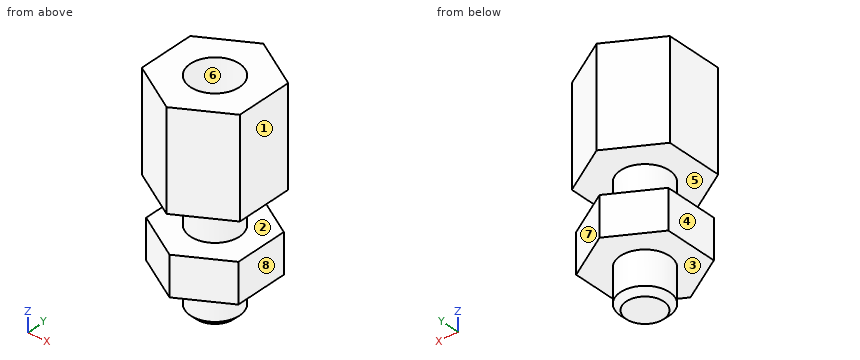
from build123d import *

# Parameters (mm, degrees)
F1_DEPTH = 5
F2_R     = 1.25
F3_DEPTH = 6
F4_R     = 1.25
F5_DEPTH = 2.5
F6_SIZE  = 0.3
F8_R     = 1.25
F9_DEPTH = 2


with BuildPart() as f1:
    # F0 (on Top) → F1 (new body)
    with BuildSketch(Plane.XY):
        Polygon((2.5, 1.443376), (0, 2.886751), (-2.5, 1.443376), (-2.5, -1.443376), (0, -2.886751), (2.5, -1.443376), align=None)
    extrude(amount=-F1_DEPTH)

    # F2 (on face) → F3 (join)
    with BuildSketch(Plane(origin=(0, 0, -5), x_dir=(1, 0, 0), z_dir=(0, 0, -1))):
        Circle(F2_R)
    extrude(amount=F3_DEPTH)

    # F4 (on face) → F5 (cut)
    with BuildSketch(Plane.XY):
        Circle(F4_R)
    extrude(amount=-F5_DEPTH, mode=Mode.SUBTRACT)

    # F6
    f6_edges = [f1.edges().sort_by_distance(p)[0] for p in [
        (-1.25, 0, -11),
    ]]
    chamfer(f6_edges, length=F6_SIZE)

    # F8 (on offset) → F9 (join)
    with BuildSketch(Plane(origin=(0, 0, -7), x_dir=(1, 0, 0), z_dir=(0, 0, -1))):
        Polygon((0, 2.713546), (-2.35, 1.356773), (-2.35, -1.356773), (0, -2.713546), (2.35, -1.356773), (2.35, 1.356773), align=None)
        Circle(F8_R, mode=Mode.SUBTRACT)
    extrude(amount=F9_DEPTH)


solid = f1.part
Could you check a few things on this model? Use its own coordinates, in mm. Face numbers are marked on the shaded views. A direction names the side the tool comes from. Coordinates: 2 decimals unless noted, no trailing zeros. Order: outer loops, then holes, each group sorted by start corner. A loop starts at its lowest first (then second) coordinate and runs counter-clockwise, first axis right, second up. Notation, with made-up numbers: (30.25, 12.25) -> (37.25, 12.25) arc R23 ccw to (37.25, 29.25) -> close; hole circle Ø3 at (88.5, -1). An arc over 180 degrees is marked (long way). One line per question, with ' | ' between items.
Q1. If I drill on L1, parallel to Z at x = 0.2, y = 1.3; L2, parallel to Y at x = 0.3, z = -4.5; L3, parallel to Z at x = -0.1, y = 0.05, over which ranges is the centre line in solid material (lowest first)?
Return value:
L1: -9 to -7, -5 to 0 | L2: -2.71 to 2.71 | L3: -11 to -2.5
Q2. Imagine slicing it at B-B on z = -7.5. Please give me the cut outline in (x, y), and give its area (3 significant figures).
Return value:
outline: (-2.35, -1.36) -> (0, -2.71) -> (2.35, -1.36) -> (2.35, 1.36) -> (0, 2.71) -> (-2.35, 1.36) -> close | area: 19.1 mm²
Q3. Imagine slicing it at C-C on y = 0. Please give me the cut outline in (x, z), and give its area (3 significant figures).
Return value:
outline: (-2.5, -5) -> (-1.25, -5) -> (-1.25, -7) -> (-2.35, -7) -> (-2.35, -9) -> (-1.25, -9) -> (-1.25, -10.7) -> (-0.95, -11) -> (0.95, -11) -> (1.25, -10.7) -> (1.25, -9) -> (2.35, -9) -> (2.35, -7) -> (1.25, -7) -> (1.25, -5) -> (2.5, -5) -> (2.5, 0) -> (1.25, 0) -> (1.25, -2.5) -> (-1.25, -2.5) -> (-1.25, 0) -> (-2.5, 0) -> close | area: 38.1 mm²
Q4. Imagine slicing it at A-A on y = -2.4. Please give me the cut outline in (x, z).
Return value:
outline: (-0.84, -5) -> (0.84, -5) -> (0.84, 0) -> (-0.84, 0) -> close; (-0.54, -9) -> (0.54, -9) -> (0.54, -7) -> (-0.54, -7) -> close
Q5. I'm going to push flat-ended pins straight in: P1, Ø1.6, axis at y = 0, z = -8.5, coming from the -X side; P2, Ø0.8, axis at x = -0.5, y = 0.5, coming from the +Z side; P3, Ø2, axis at y = 0, z = -9, coming from the +X side. Where does each tip first touch, or does it pass through?
Return value:
P1: x = -2.35 | P2: z = -2.5 | P3: x = 2.35
Q6. Thinking about a two-plate mould opening in Z: for the marked faces 1, 2 and 3, which applies, pulls with the +Z half, pulls with the -Z half, needs draft (parallel to the pull), parting line crosses it, or undercut?
Return value:
face 1: needs draft | face 2: undercut | face 3: pulls with the -Z half
Q7. On a 3-axis mill with a long thin cutter (end or side, diameter ignored), from which of +Z, -Z, +X, -X, +Y, -Y can I reach the whole of each face in a straight line? I mean the marked faces 4, 5, 6, 7 and 8. Say none if no direction works.
Return value:
face 4: -Z, -X, +Y, -Y | face 5: none | face 6: +Z | face 7: -Z, +X, +Y | face 8: -Z, +X, +Y, -Y
Q8. Imagine slicing it at D-D on x = -1.85. Please give me the cut outline in (y, z), and give its area (3 significant figures).
Return value:
outline: (-1.82, -5) -> (1.82, -5) -> (1.82, 0) -> (-1.82, 0) -> close; (-1.65, -9) -> (1.65, -9) -> (1.65, -7) -> (-1.65, -7) -> close | area: 24.8 mm²
